Study the drawing (mm; zero at the part's minimum x, y, z) and answer. A direction names the side the tool comes from. Coordinates: 2 decimals unless noted, no trailing zeros. Order: outer loops, then holes, each group sorted by start corner. A loop starts at its lowest first (then second) coordinate and runs counter-clockwise, first axis right, second up.
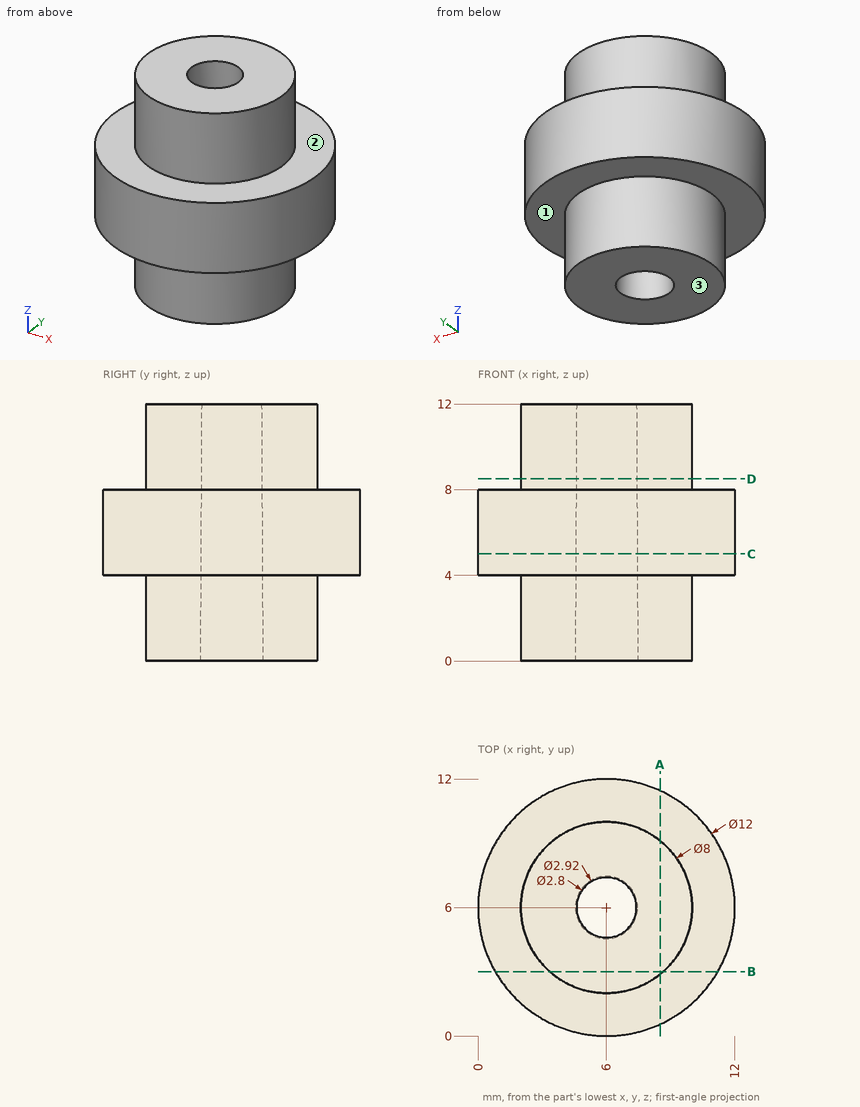
1) A cutting plane is placed at A-A, the plane x = 8.5. Determine the outline of the cut face in (y, z), and give its area (3 significant figures).
A:
outline: (0.55, 4) - (2.88, 4) - (2.88, 0) - (9.12, 0) - (9.12, 4) - (11.45, 4) - (11.45, 8) - (9.12, 8) - (9.12, 12) - (2.88, 12) - (2.88, 8) - (0.55, 8) - close
area: 93.6 mm2
2) Flat-ended cylindrical pins translate along their axes: pin 1 Ø4 at (x, z) = (9.5, 2.5) entering from -Y; pin 2 Ø1.5 at (x, y) = (5, 2) entering from +Z; pin 3 Ø3 at (x, z) = (9.5, 5) entering from +Y; pin 4 Ø4 at (x, z) = (1.5, 7.5) entering from -Y. Find the tip coordinate at first contact, or state that the pin passes through.
A:
pin 1: stops at y = 0.41
pin 2: stops at z = 12
pin 3: stops at y = 11.66
pin 4: stops at y = 0.55
3) A cutting plane is placed at B-B, the plane y = 3. Determine the outline of the cut face in (x, z), and give its area (3 significant figures).
A:
outline: (0.8, 4) - (3.35, 4) - (3.35, 0) - (8.65, 0) - (8.65, 4) - (11.2, 4) - (11.2, 8) - (8.65, 8) - (8.65, 12) - (3.35, 12) - (3.35, 8) - (0.8, 8) - close
area: 83.9 mm2
4) Which of the six approach directions +Z, -Z, +X, -X, +Y, -Y give full straight-line access (tool end or side, diameter ignored) to the marked faces 1, 2 and 3?
A:
face 1: -Z
face 2: +Z
face 3: -Z, +X, -X, +Y, -Y
5) Straight lines are drawn through the part: line 1 (Z direction, x = 7.75, y = 11.5); line 2 (Y direction, x = 7, z = 10.75); line 3 (Y direction, x = 5.25, z = 5). For each, find the intervals that lie inside material, in ascending order.
A:
line 1: z = 4 to 8
line 2: y = 2.13 to 5.01, 6.99 to 9.87
line 3: y = 0.05 to 4.78, 7.22 to 11.95
6) A cutting plane is placed at D-D, the plane z = 8.5. Determine the outline of the cut face in (x, y) (1 decimal).
A:
outline: circle Ø8 at (6, 6); hole circle Ø2.8 at (6, 6)
7) A cutting plane is placed at C-C, the plane z = 5. Determine the outline of the cut face in (x, y) (3 decimals), and give its area (3 significant figures).
A:
outline: circle Ø12 at (6, 6); hole circle Ø2.87 at (6, 6)
area: 107 mm2
